Input: dimensioned drawing with shaded views. Units: mm. Origin: part minimum x, y, z. A direction names the side the tool comes from. Give positions to 0.01 mm unless a question says otherwise; leave off trailing zeros. Write each loop counter-clockwise with the first axis right and the second up, starting at its lowest first coordinate (ties: lowest second). Pieces come first, ordered by that corner, then holes. Notation, with made-up numbers: (-40, -27) - (9, -27) arc R24 cw to (9, 0) - close; hole circle Ø1 at (14.25, 49.25). An arc over 180 degrees is marked (long way). Answer as a JSON object with one key per item and string values. Group by question number.
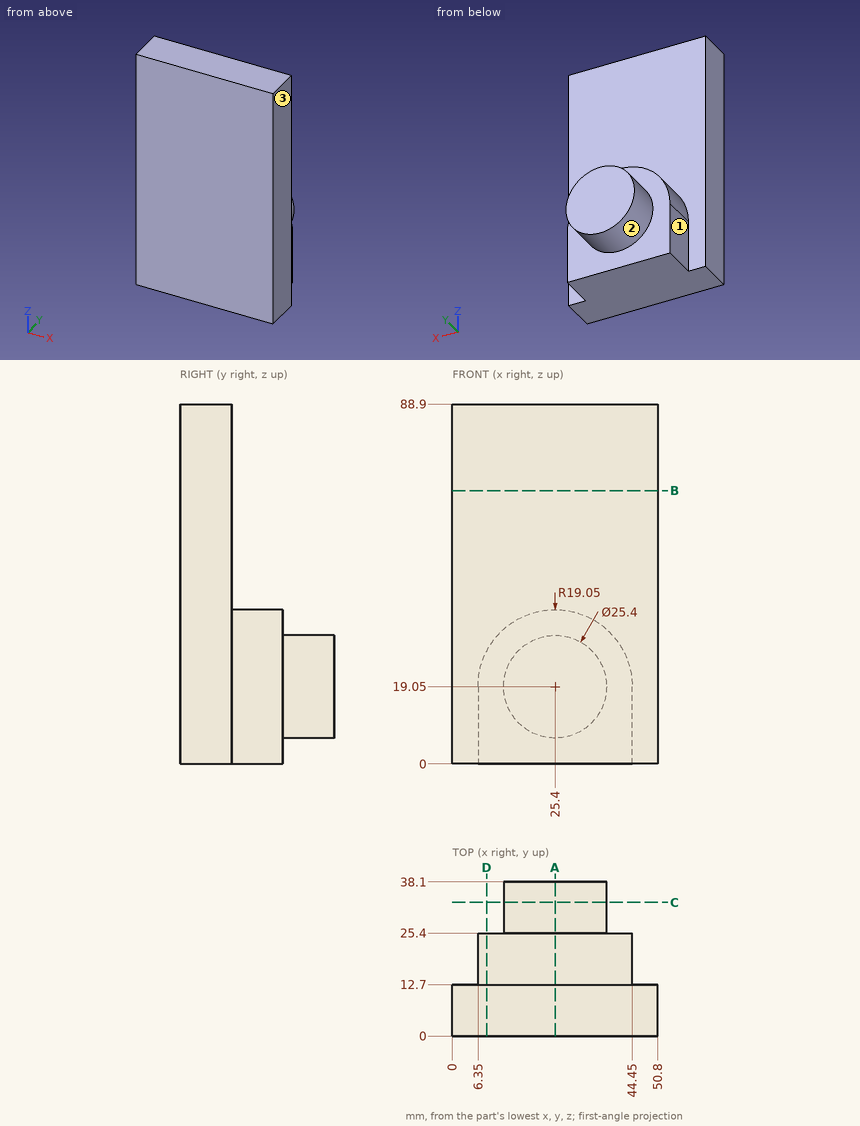
Q1. First-contact query: pin 1 Ø5 at (x, y) = (34, 29) entering from +Z; pin 2 Ø2 at (y, z) = (14, 23.5) entering from -X (3 decimals); pin 3 Ø1.5 at (y, z) = (17.5, 33.5) entering from +X. Flat tips, straight axial feed; report the tip coordinate or a pass-through.
Q2. Section C-C on y = 33. Return the cut outline in (x, z).
Q3. Section D-D on x = 8.5. Return the cut outline in (y, z), then the cut area to 3 significant figures.
Q4. Section A-A on x = 25.4. Return the cut outline in (y, z), then the cut area to 3 significant figures.
Q5. Section B-B on z = 67.5. Return the cut outline in (x, y), then the cut area to 3 significant figures.
Q6. Ray query, probe 1 along Y at (x, z) = (42, 58.5); probe 2 along Y at (x, z) = (44, 22); probe 3 along Z at (x, y) = (25, 19). Return the intervals inside material, ascending. Write a range as [from, to].
Q7. Reachability of the marked faces 1, 2 and 3 from +Z, -Z, +X, -X, +Y, -Y: full face, straight path, thin tool, end or side. Return the list, or none.
Taken from the geometry:
{
 "1": {"pin 1": "stops at z = 30.19", "pin 2": "stops at x = 6.665", "pin 3": "stops at x = 38.64"},
 "2": {"outline": "circle Ø25.4 at (25.4, 19.05)"},
 "3": {"outline": "(0, 0) - (25.4, 0) - (25.4, 27.84) - (12.7, 27.84) - (12.7, 88.9) - (0, 88.9) - close", "area": "1,480 mm²"},
 "4": {"outline": "(0, 0) - (25.4, 0) - (25.4, 6.35) - (38.1, 6.35) - (38.1, 31.75) - (25.4, 31.75) - (25.4, 38.1) - (12.7, 38.1) - (12.7, 88.9) - (0, 88.9) - close", "area": "1,940 mm²"},
 "5": {"outline": "(0, 0) - (50.8, 0) - (50.8, 12.7) - (0, 12.7) - close", "area": "645 mm²"},
 "6": {"probe 1": "y = [0, 12.7]", "probe 2": "y = [0, 25.4]", "probe 3": "z = [0, 38.1]"},
 "7": {"face 1": "+Z, -Z, -X, +Y", "face 2": "+Y", "face 3": "+Z, -Z, +X, +Y, -Y"}
}
